The listing builds one solid part. Answer for the finished solid, in the listing's coordinates (mm). A direction names the side the tool comes from. Coordinates: 2 decimals unless noted, no trailing zeros. Order: outer loops, then holes, each group sorted by start corner. A loop starts at its lowest first (then second) coordinate and runs counter-clockwise, first axis right, second up.
```python
from build123d import *

# Parameters (mm, degrees)
SKETCH_1_R               = 6.11
SKETCH_1_R_2             = 2.5
EXTRUDE_1_DEPTH          = 16
SKETCH_1_3_R             = 8
SKETCH_1_3_R_2           = 6.11
EXTRUDE_2_DEPTH          = 8
EXTRUDE_START            = -1
SKETCH_2_R               = 8
SKETCH_2_R_2             = 6.11
EXTRUDE_3_DEPTH          = 1
CUT_EXTRUDE_5_DEPTH      = 7
PATTERN_CIRCULAR_1_COUNT = 20


with BuildPart() as part:
    # Эскиз1 → Бобышка-Вытянуть1 (new body)
    with BuildSketch(Plane.XY):
        Circle(SKETCH_1_R)
        Circle(SKETCH_1_R_2, mode=Mode.SUBTRACT)
    extrude(amount=EXTRUDE_1_DEPTH)

    # Эскиз1<3> → Бобышка-Вытянуть2 (add)
    with BuildSketch(Plane.XY):
        Circle(SKETCH_1_3_R)
        Circle(SKETCH_1_3_R_2, mode=Mode.SUBTRACT)
    extrude(amount=EXTRUDE_2_DEPTH)

    # Эскиз2 → Бобышка-Вытянуть3 (add)
    with BuildSketch(Plane.XY.offset(16).offset(EXTRUDE_START)):
        Circle(SKETCH_2_R)
        Circle(SKETCH_2_R_2, mode=Mode.SUBTRACT)
    extrude(amount=EXTRUDE_3_DEPTH)

    # Эскиз3 → Вырез-Вытянуть5 (cut)
    with BuildSketch(Plane.XY.offset(8)):
        with BuildLine():
            Line((-0.3, 5), (0.3, 5))
            Line((0.3, 5), (0.70385757, 6.109589554))
            ThreePointArc((0.70385757, 6.109589554), (0, 6.15), (-0.70385757, 6.109589554))
            Line((-0.70385757, 6.109589554), (-0.3, 5))
        make_face()
    cut_extrude_5 = extrude(amount=CUT_EXTRUDE_5_DEPTH, mode=Mode.SUBTRACT)

    # Круговой массив1: Вырез-Вытянуть5 ×20 about axis
    pattern_circular_1_axis = Axis((0, 0, 0), (0, 0, 1))
    for i in range(1, PATTERN_CIRCULAR_1_COUNT):
        add(cut_extrude_5.rotate(pattern_circular_1_axis, i * 360 / PATTERN_CIRCULAR_1_COUNT), mode=Mode.SUBTRACT)


solid = part.part
```
(1) Find section A-A (y = 0). Write down the section's boundary in (x, z).
(2) The mould has two halves that part along Z. Classify faces 5 (the face through (-2.18, -5.11, 11.45)), 6 (the face through (2.19, -5.12, 11.45)): released by +Z, released by -Z, zero draft, split by the parting line, or undercut.
(3) Each of these flat-tipped pins is pushed along its axis until it touches: pin 1 Ø1 at (y, z) = (2.5, 13) entering from +X; pin 2 Ø5 at (y, z) = (3.5, 4.5) entering from +X; pin 3 Ø4 at (x, z) = (-6, 11.5) entering from -Y. Where does it stop, or does it pass through?
(4) Consider line 1 (Z direction, x = -3, y = -4.25); line 2 (Y direction, x = 0, z = 4.5); line 3 (Y direction, x = 0, z = 13). Determine where each line is inside the solid, lowest interval first.
(5) For faces 1 (the face through (4.183, -3.647, 11.451)), 2 (the face through (0.492, 5.528, 11.451)), 3 (the face through (-5.12, -2.19, 11.45)), 4 (the face through (-2.85, 4.76, 11.45)), determine the directions among +Z, -Z, +X, -X, +Y, -Y from which every point of the face is accessible in a straight line to the end or side of a thin tool.
(6) Find section C-C (z = 4). Write down the section's boundary in (x, y).
Findings below:
1. outline: (-8, 0) - (-2.5, 0) - (-2.5, 16) - (-8, 16) - (-8, 15) - (-5, 15) - (-5, 8) - (-8, 8) - close; (2.5, 0) - (8, 0) - (8, 8) - (5, 8) - (5, 15) - (8, 15) - (8, 16) - (2.5, 16) - close
2. face 5: undercut
2. face 6: undercut
3. pin 1: stops at x = 5.56
3. pin 2: stops at x = 7.94
3. pin 3: stops at y = -4.51
4. line 1: z = 0 to 8, 15 to 16
4. line 2: y = -8 to -2.5, 2.5 to 8
4. line 3: y = -5 to -2.5, 2.5 to 5
5. face 1: +X
5. face 2: +Y
5. face 3: -X
5. face 4: none
6. outline: circle Ø16 at (0, 0); hole circle Ø5 at (0, 0)
